from build123d import *

# Parameters (mm, degrees)
EXTRUDE_DEPTH   = 8
CHAMFER_SIZE    = 1
CHAMFER001_SIZE = 1


with BuildPart() as part:
    # Sketch → Extrude (new body)
    with BuildSketch(Plane.XZ):
        Polygon((-1.25, 10), (1.25, 10), (4, 7.25), (-4, 7.25), align=None)
    extrude(amount=EXTRUDE_DEPTH)

    # Chamfer
    chamfer_edges = [part.edges().sort_by_distance(p)[0] for p in [
        (0, 0, 10),
    ]]
    chamfer(chamfer_edges, length=CHAMFER_SIZE)

    # Chamfer001
    chamfer001_edges = [part.edges().sort_by_distance(p)[0] for p in [
        (0, -8, 10),
    ]]
    chamfer(chamfer001_edges, length=CHAMFER001_SIZE)


solid = part.part
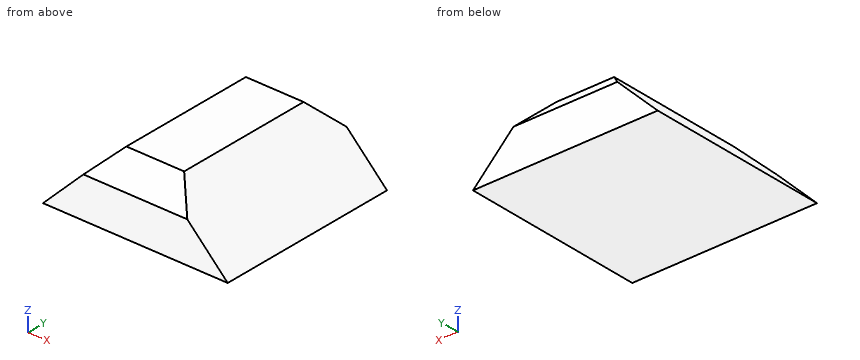
Input: part model. Units: mm. Frame: model coordinates. Coordinates: 2 decimals unless noted, no trailing zeros. Order: outer loops, then holes, each group sorted by start corner. A loop starts at its lowest first (then second) coordinate and runs counter-clockwise, first axis right, second up. Notation, with made-up numbers: M 81.25,81 L 112.25,81 A34 ccw 112.25,116 Z; hole C 28.5,29.25 d10. An arc over 180 degrees is marked long. Write item = value, one per line. Start each with the question number.
(1) Line query: line 1 along Z through (x, y) = (-1.75, -5.25); line 2 along X through (y, z) = (-5.75, 8.9); line 3 along Z through (x, y) = (-1.5, -5). Output: solid intervals per line, ascending. Write a range as [from, to].
(2) Section B-B on z = 8.7. Output: boundary loops of the cut face in (x, y).
(3) Section C-C on y = -6.75. Output: boundary loops of the cut face in (x, z), and give its area (3 significant figures).
(4) Section A-A on x = -1.5. Output: boundary loops of the cut face in (y, z), and give its area (3 significant figures).
(5) Section D-D on x = 0.5. Output: boundary loops of the cut face in (y, z).
Result set:
q1.line_1 = [7.25, 9.5]
q1.line_2 = [-2.35, 2.35]
q1.line_3 = [7.25, 9.75]
q2.outline = M -2.55,-8 L 2.55,-8 L 2.55,0 L -2.55,0 Z
q3.outline = M -4,7.25 L 4,7.25 L 1.25,10 L -1.25,10 Z
q3.area = 14.4 mm²
q4.outline = M -8,7.25 L 0,7.25 L 0,9 L -0.75,9.75 L -7.25,9.75 L -8,9 Z
q4.area = 19.4 mm²
q5.outline = M -8,7.25 L 0,7.25 L 0,9 L -1,10 L -7,10 L -8,9 Z
